from build123d import *

# Parameters (mm, degrees)
F0_R     = 12.5
F1_DEPTH = 50
F2_SIZE  = 2.49999


# Not quite as in the source:
# - a fillet or chamfer is up to 0.001 mm smaller than in the source, because OpenCascade refuses the exact size


with BuildPart() as f1:
    # F0 (on Top) → F1 (new body, symmetric)
    with BuildSketch(Plane.XY):
        with BuildLine():
            ThreePointArc((-50, -47.5), (-49.267766953, -49.267766953), (-47.5, -50))
            Line((-47.5, -50), (47.5, -50))
            ThreePointArc((47.5, -50), (49.267766953, -49.267766953), (50, -47.5))
            Line((50, -47.5), (50, 47.5))
            ThreePointArc((50, 47.5), (49.267766953, 49.267766953), (47.5, 50))
            Line((47.5, 50), (-47.5, 50))
            ThreePointArc((-47.5, 50), (-49.267766953, 49.267766953), (-50, 47.5))
            Line((-50, 47.5), (-50, -47.5))
        make_face()
        Circle(F0_R, mode=Mode.SUBTRACT)
    extrude(amount=F1_DEPTH, both=True)

    # F2 (size 2.5 in the source; OpenCascade refuses exactly that, so slightly less here)
    f2_edges = [f1.edges().sort_by_distance(p)[0] for p in [
        (50, 0, 50),
        (0, -50, 50),
        (-50, 0, 50),
        (0, 50, 50),
        (50, 0, -50),
        (0, 50, -50),
    ]]
    chamfer(f2_edges, length=F2_SIZE)


solid = f1.part
Build history of the part. All positions in model axes, mm. Give positions to 0.01 mm unless a question says otherwise; leave off trailing zeros. Order: outer loops, then holes, each group sorted by start corner. A loop starts at its lowest first (then second) coordinate and runs counter-clockwise, first axis right, second up. Notation, with made-up numbers: M 36,1.25 L 43,1.25 A16 ccw 43,16.25 Z; hole C 56.5,76 d7. An arc over 180 degrees is marked long. Put each result on its own line as item: value.
Item 1: Cut at A-A on y = 0. Write the cut outline in (x, z), then the cut area to 3 significant figures.
Results are:
outline: M -50,-47.5 L -47.5,-50 L -12.5,-50 L -12.5,50 L -47.5,50 L -50,47.5 Z; M 12.5,-50 L 47.5,-50 L 50,-47.5 L 50,47.5 L 47.5,50 L 12.5,50 Z
area: 7,490 mm2
Item 2: Cut at C-C on z = 8.5. Write the cut outline in (x, y).
Results are:
outline: M -50,-47.5 A2.5 ccw -47.5,-50 L 47.5,-50 A2.5 ccw 50,-47.5 L 50,47.5 A2.5 ccw 47.5,50 L -47.5,50 A2.5 ccw -50,47.5 Z; hole C 0,0 d25
Item 3: Wall check: probe 1 along Y at (x, z) = (0, -2); probe 2 along X at (y, z) = (10.5, 17). Give the ranges that are in metal, low to high.
Results are:
probe 1: -50 to -12.5, 12.5 to 50
probe 2: -50 to -6.78, 6.78 to 50
Item 4: Pull direction Y, two halves, no side cores. Call faces 1 (the face through (-11, 11, -50)), 2 (the face through (-1, -50, 1)), 3 (the face through (11.923, 3.755, -0.7)), 4 (the face through (1, 50, 1)): +Y half, -Y half, draft (parallel to the pull), parting line (faces both ways), or undercut.
Results are:
face 1: draft
face 2: -Y half
face 3: undercut
face 4: +Y half
